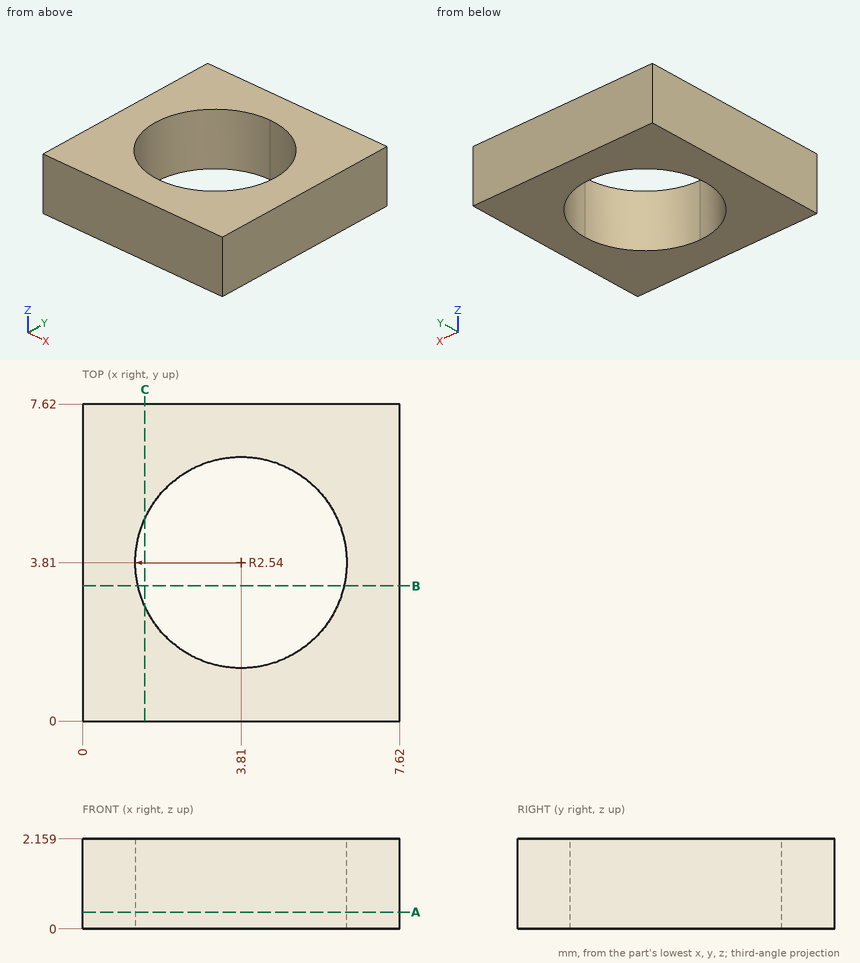
Part print with two shaded views. Sizes in mm from the minimum x, y, z corner. Coordinates: 2 decimals unless noted, no trailing zeros. Write each loop counter-clockwise with the first axis right and the second up, starting at its lowest first coordinate (ties: lowest second). Pieces come first, ordered by that corner, then holes. Notation, with made-up numbers: (86, 78) - (104, 78) arc R8 cw to (104, 91) - close; hole circle Ø9 at (32, 52.25). An arc over 180 degrees is marked (long way). Use a Markdown table: item, result. Add a question column.
Item 1: Drill centre lines: line 1 along X through (y, z) = (3.75, 2.1); line 2 along Y through (x, z) = (2.75, 1.3); line 3 along Y through (x, z) = (4.5, 1.7). Where is each one in solid material? Low to high.
Item 2: Band-saw the part on C-C, the plane x = 1.5. Write the cut outline in (y, z).
Item 3: Band-saw the part on B-B, the plane y = 3.25. Write the cut outline in (x, z).
Item 4: Band-saw the part on A-A, the plane z = 0.4. Write the cut outline in (x, y), and give its area (3 significant figures).
A:
| question | item | result |
|---|---|---|
| 1 | line 1 | x = 0 to 1.27, 6.35 to 7.62 |
| 1 | line 2 | y = 0 to 1.5, 6.12 to 7.62 |
| 1 | line 3 | y = 0 to 1.37, 6.25 to 7.62 |
| 2 | outline | (0, 0) - (2.75, 0) - (2.75, 2.16) - (0, 2.16) - close; (4.87, 0) - (7.62, 0) - (7.62, 2.16) - (4.87, 2.16) - close |
| 3 | outline | (0, 0) - (1.33, 0) - (1.33, 2.16) - (0, 2.16) - close; (6.29, 0) - (7.62, 0) - (7.62, 2.16) - (6.29, 2.16) - close |
| 4 | outline | (0, 0) - (7.62, 0) - (7.62, 7.62) - (0, 7.62) - close; hole (3.81, 6.35) arc R2.54 ccw (long way) to (6.35, 3.81) arc R2.54 ccw to start |
| 4 | area | 37.8 mm² |
